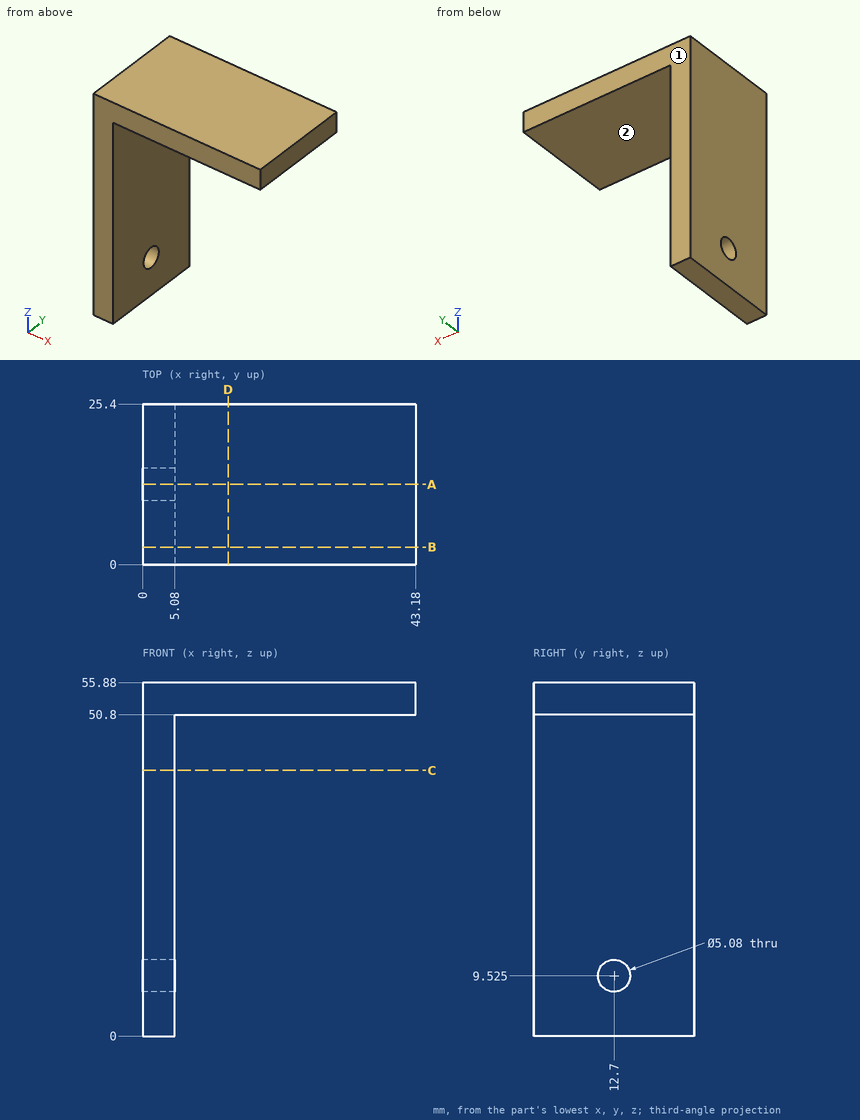
Source: three-view drawing plus pictorial views. Frame: mm from the lowest corner of the part. A direction names the side the tool comes from. Give positions to 0.01 mm unless a question says otherwise; leave off trailing zeros. Loops run counter-clockwise (first coordinate to the right, second up) from the corner with the lowest first, then second, coordinate; pieces in that order, holes last. Notation, with made-up numbers: (-5, -13.75) -> (1, -13.75) arc R24 cw to (1, 8.25) -> close; hole circle Ø5 at (12.25, 20). An arc over 180 degrees is marked (long way). Use a Markdown table: item, result. Add a question column.
(1) Section query C-C (z = 42). Output: boundary loops of the cut face in (x, y).
(2) Access query for the marked faces 1 and 2. Directions: +Z, -Z, +X, -X, +Y, -Y. A direction counts if a zero-diameter tool reaches every point of the face in a straight line with its end or side. Return the directions, or none.
(3) First-contact query: pin 1 Ø10 at (x, z) = (16, 43) entering from +Y; pin 2 Ø7.5 at (y, z) = (7.5, 23.5) entering from +X; pin 3 Ø4 at (x, y) = (30, 3.5) entering from -Z. Flat tips, straight axial feed; report the tip coordinate or a pass-through.
(4) Ray query, line 1 (Z direction, x = 2.95, y = 12.7) (3 decimals); line 2 (X direction, y = 17.75, z = 26); line 3 (Z direction, x = 40.5, y = 24.5). Return the intervals inside material, ascending.
(5) Section query D-D (x = 13.5). Output: boundary loops of the cut face in (y, z), then the cut area to 3 significant figures.
(6) Section query B-B (y = 2.75). Output: boundary loops of the cut face in (x, z).
(7) Section query A-A (y = 12.7). Output: boundary loops of the cut face in (x, z) (3 decimals), then the cut area to 3 significant figures.
Checked values:
| question | item | result |
|---|---|---|
| 1 | outline | (0, 0) -> (5.08, 0) -> (5.08, 25.4) -> (0, 25.4) -> close |
| 2 | face 1 | +Z, -Z, +X, -X, +Y |
| 2 | face 2 | -Z, +X, +Y, -Y |
| 3 | pin 1 | through |
| 3 | pin 2 | x = 5.08 |
| 3 | pin 3 | z = 50.8 |
| 4 | line 1 | 0 to 6.985, 12.065 to 55.88 |
| 4 | line 2 | 0 to 5.08 |
| 4 | line 3 | 50.8 to 55.88 |
| 5 | outline | (0, 50.8) -> (25.4, 50.8) -> (25.4, 55.88) -> (0, 55.88) -> close |
| 5 | area | 129 mm^2 |
| 6 | outline | (0, 0) -> (5.08, 0) -> (5.08, 50.8) -> (43.18, 50.8) -> (43.18, 55.88) -> (0, 55.88) -> close |
| 7 | outline | (0, 0) -> (5.08, 0) -> (5.08, 6.985) -> (0, 6.985) -> close; (0, 12.065) -> (5.08, 12.065) -> (5.08, 50.8) -> (43.18, 50.8) -> (43.18, 55.88) -> (0, 55.88) -> close |
| 7 | area | 452 mm^2 |
